```python
from build123d import *

# Parameters (mm, degrees)
BOSS_EXTRUDE1_DEPTH = 20
CUT_EXTRUDE1_DEPTH  = 20


with BuildPart() as part:
    # Sketch2 → Boss-Extrude1 (new body)
    with BuildSketch(Plane(origin=(0, 0, 0), x_dir=(1, 0, 0), z_dir=(0, 1, 0))):
        Polygon((0, 0), (50, 0), (50, -50), (45, -50), (45, -30), (20, -30), (20, -5), (0, -5), align=None)
    extrude(amount=BOSS_EXTRUDE1_DEPTH)

    # Sketch3 → Cut-Extrude1 (cut)
    with BuildSketch(Plane(origin=(0, 20, 0), x_dir=(1, 0, 0), z_dir=(0, 1, 0))):
        Polygon((39.341240981, -22.493572362), (43.660244521, -14.987161207), (39.31900354, -7.493588845), (30.658759019, -7.506427638), (26.339755479, -15.012838793), (30.68099646, -22.506411155), align=None)
    extrude(amount=-CUT_EXTRUDE1_DEPTH, mode=Mode.SUBTRACT)


solid = part.part
```
Model file for the job. Use its own axes, mm. A direction names the side the tool comes from. Give positions to 0.01 mm unless a question says otherwise; leave off trailing zeros. Order: outer loops, then holes, each group sorted by start corner. A loop starts at its lowest first (then second) coordinate and runs counter-clockwise, first axis right, second up.
1) Wall check: probe 1 along Z at (x, y) = (31, 15); probe 2 along Z at (x, y) = (3, 9); probe 3 along X at (y, z) = (1.75, 16.5). Give the ranges that are in metal, low to high.
2) Saw through at D-D, the plane x = 22. Write the cut outline in (y, z).
3) Saw through at A-A, the plane y = 2.75. Write the cut outline in (x, z).
4) 3-axis set-ups, long thin cutter, end or side, ignore diameter. For faces 1 (the flat face through (28.53, 10.14, 11.21)), 2 (the flat face through (0, 10, 3)), 3 (the flat face through (45, 10, 40)): which of +Z, -Z, +X, -X, +Y, -Y reach the whole face in a straight line?
5) Mould opens along Z. For faces 4 (the flat face through (27, 20, 12)), 5 (the flat face through (33, 10, 30)), 6 (the flat face through (41.52, 10.14, 11.29)) say: +Z half, -Z half, draft (parallel to the pull), parting line (faces both ways), or undercut.
6) Saw through at B-B, the plane z = 13. Write the cut outline in (x, y), then the cut area to 3 significant figures.
7) Saw through at C-C, the plane x = 41. Write the cut outline in (y, z), then the cut area to 3 significant figures.
8) Pin check, flat tips, straight feed: pin 1 (10 mm diameter, centred on x = 28.5, y = 17, fed in from -Z); pin 2 (10 mm diameter, centred on y = 14.5, z = 25.5, fed in from -X); pin 3 (1 mm diameter, centred on x = 30.5, y = 12.5, fed in from +Z); pin 4 (10 mm diameter, centred on y = 11.5, z = 38.5, fed in from -X). Stop position of each tip, or through.
Computed:
1. probe 1: z = 0 to 7.51, 22.51 to 30
1. probe 2: z = 0 to 5
1. probe 3: x = 20 to 27.2, 42.79 to 50
2. outline: (0, 0) - (20, 0) - (20, 30) - (0, 30) - close
3. outline: (0, 0) - (50, 0) - (50, 50) - (45, 50) - (45, 30) - (20, 30) - (20, 5) - (0, 5) - close; hole (26.34, 15.01) - (30.66, 7.51) - (39.32, 7.49) - (43.66, 14.99) - (39.34, 22.49) - (30.68, 22.51) - close
4. face 1: +Y, -Y
4. face 2: +Z, -Z, -X, +Y, -Y
4. face 3: +Z, -X, +Y, -Y
5. face 4: draft
5. face 5: +Z half
5. face 6: undercut
6. outline: (20, 0) - (27.5, 0) - (27.5, 20) - (20, 20) - close; (42.51, 0) - (50, 0) - (50, 20) - (42.51, 20) - close
6. area: 300 mm2
7. outline: (0, 0) - (20, 0) - (20, 10.4) - (0, 10.4) - close; (0, 19.61) - (20, 19.61) - (20, 30) - (0, 30) - close
7. area: 416 mm2
8. pin 1: stops at z = 0
8. pin 2: stops at x = 20
8. pin 3: stops at z = 30
8. pin 4: stops at x = 45
